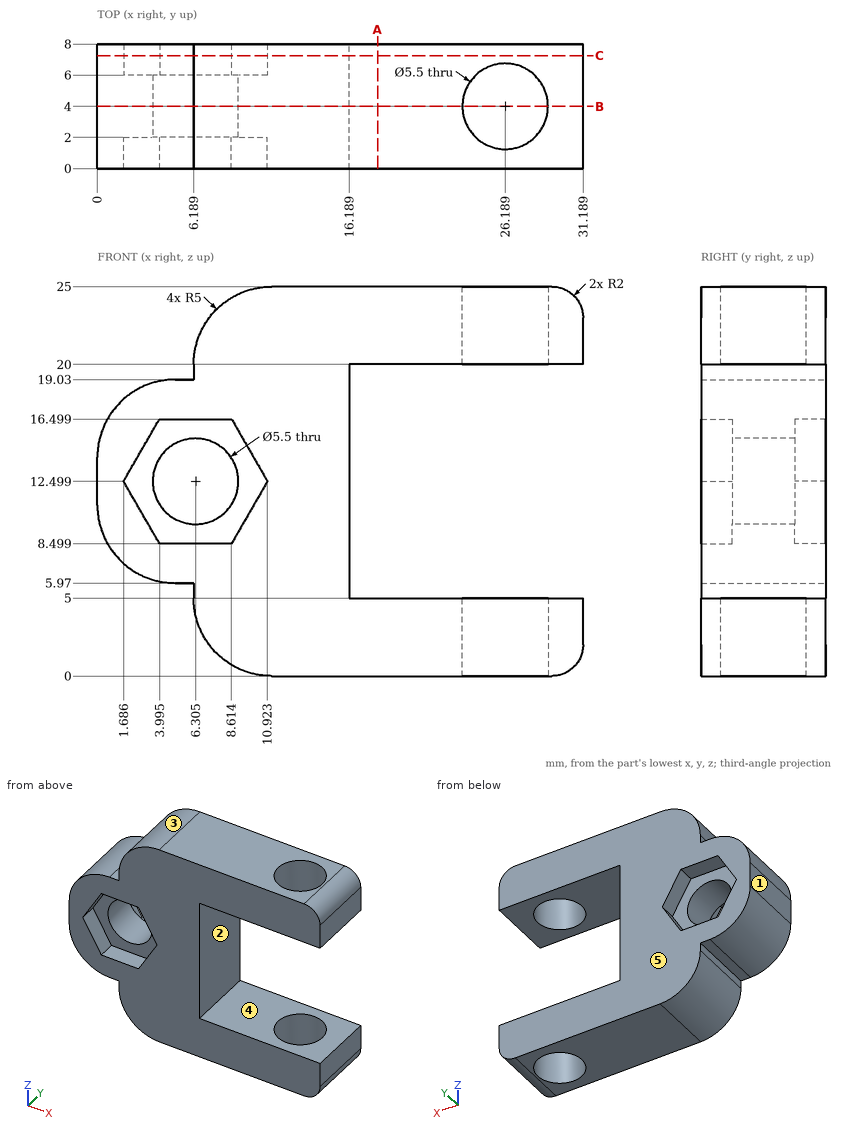
Study the drawing (mm; zero at the part's minimum x, y, z) and answer. A direction names the side the tool comes from. Coordinates: 2 decimals unless noted, no trailing zeros. Write each loop counter-clockwise with the first axis right and the second up, starting at its lowest first coordinate (ties: lowest second). Pieces come first, ordered by that corner, then holes. Notation, with made-up numbers: M 55,71 L 74,71 A16 cw 74,98 Z; hole C -12,24.25 d5. An arc over 180 degrees is marked long. Use a Markdown table: item, result. Add a question column.
1. Which of the six approach directions +Z, -Z, +X, -X, +Y, -Y give full straight-line access (tool end or side, diameter ignored) to the marked faces 4 and 5?
2. For a pull along Z with two mould halves and no side action, classify the marked faces 1, 2 and 3 as +Z half, -Z half, draft (parallel to the pull), parting line (faces both ways), or undercut.
3. Section C-C (y = 7.25) is taken. Give the vertices of the cut face in (x, z) (1 decimal), plus the area to 3 significant figures.
4. Section B-B (y = 4) is taken. Count the separate pieces of the cut face and the enclosed holes in it, plus the area to 3 significant figures.
5. Given P1, Ø0.6, axis at x = 5.5, y = 4, coming from the -Z side; P2, Ø4, axis at y = 2.5, z = 9, coming from the +X side; P3, Ø1, axis at x = 5.5, y = 2.5, coming from the +Z side, each flat-ended and moving along its own axis, determine where each tip first touches the part or whether it passes through.
6. Section A-A (x = 18) is taken. Give the vertices of the cut face in (y, z).
7. Straight lines are drawn through the part: line 1 along Z through (x, y) = (18.5, 6.5); line 2 along X through (y, z) = (4.25, 13.25); line 3 along Z through (x, y) = (4, 5.25). For each, find the intervals that lie inside material, in ascending order. Write a range as [from, to].
Data:
| question | item | result |
|---|---|---|
| 1 | face 4 | +X, +Y, -Y |
| 1 | face 5 | +Z, -Z, +X, -X, +Y |
| 2 | face 1 | draft |
| 2 | face 2 | undercut |
| 2 | face 3 | +Z half |
| 3 | outline | M 0,11 A5 ccw 5,6 L 6.2,6 L 6.2,5 A5 ccw 11.2,0 L 29.2,0 A2 ccw 31.2,2 L 31.2,5 L 16.2,5 L 16.2,20 L 31.2,20 L 31.2,23 A2 ccw 29.2,25 L 11.2,25 A5 ccw 6.2,20 L 6.2,19 L 5,19 A5 ccw 0,14 Z; hole M 1.7,12.5 L 4,8.5 L 8.6,8.5 L 10.9,12.5 L 8.6,16.5 L 4,16.5 Z |
| 3 | area | 402 mm2 |
| 4 | separate pieces | 3 |
| 4 | enclosed holes | 1 |
| 4 | area | 379 mm2 |
| 5 | P1 | stops at z = 5.97 |
| 5 | P2 | stops at x = 16.19 |
| 5 | P3 | stops at z = 19.03 |
| 6 | outline | M 0,0 L 8,0 L 8,5 L 0,5 Z; M 0,20 L 8,20 L 8,25 L 0,25 Z |
| 7 | line 1 | z = [0, 5], [20, 25] |
| 7 | line 2 | x = [0, 3.66], [8.95, 16.19] |
| 7 | line 3 | z = [6.07, 11], [14, 18.93] |
